Geometry: final body of the model. Coordinates: model frame, mm. Coordinates: 2 decimals unless noted, no trailing zeros. Write each loop counter-clockwise with the first axis right and the second up, starting at its lowest first coordinate (ties: lowest second). Pieces come first, ordered by that corner, then holes. Notation, with made-up numbers: (3.25, -31) -> (26.25, -31) arc R22 cw to (26.25, 6) -> close; hole circle Ø1 at (49.5, -17.5). An arc over 180 degrees is marked (long way). Answer as a JSON object with one key per item and string values. Group by question number.
```python
from build123d import *

# Parameters (mm, degrees)
SKETCH1_R           = 2.55
SKETCH1_R_2         = 4.5
SKETCH1_R_3         = 2.65
SKETCH1_W           = 44
SKETCH1_H           = 5
BOSS_EXTRUDE1_DEPTH = 5


with BuildPart() as part:
    # Sketch1 → Boss-Extrude1 (new body)
    with BuildSketch(Plane(origin=(0, 0, 0), x_dir=(1, 0, 0), z_dir=(0, 1, 0))):
        with BuildLine():
            Line((0, 0), (0, 33.5))
            ThreePointArc((0, 33.5), (-1.464466094, 37.035533906), (-5, 38.5))
            Line((-5, 38.5), (-31, 38.5))
            Line((-31, 38.5), (-31, 65))
            Line((-31, 65), (-564, 65))
            Line((-564, 65), (-564, -65))
            Line((-564, -65), (-524.5, -65))
            Line((-524.5, -65), (0, -65))
            Line((0, -65), (0, 0))
        make_face()
        with Locations(Location((-24.5, 33.5, 0), (0, 0, 270))):
            Circle(SKETCH1_R, mode=Mode.SUBTRACT)
        with Locations(Location((-24.5, -2.5, 0), (0, 0, 270))):
            Circle(SKETCH1_R, mode=Mode.SUBTRACT)
        with Locations(Location((-24.5, 15.5, 0), (0, 0, 270))):
            Circle(SKETCH1_R_2, mode=Mode.SUBTRACT)
        with Locations(Location((-531, -51, 0), (0, 0, 270))):
            Circle(SKETCH1_R_3, mode=Mode.SUBTRACT)
        with Locations(Location((-406, -51, 0), (0, 0, 270))):
            Circle(SKETCH1_R_3, mode=Mode.SUBTRACT)
        with Locations(Location((-281, -51, 0), (0, 0, 270))):
            Circle(SKETCH1_R_3, mode=Mode.SUBTRACT)
        with Locations(Location((-156, -51, 0), (0, 0, 270))):
            Circle(SKETCH1_R_3, mode=Mode.SUBTRACT)
        with Locations(Location((-31, -51, 0), (0, 0, 270))):
            Circle(SKETCH1_R_3, mode=Mode.SUBTRACT)
        with Locations((-472.510496642, 37)):
            Rectangle(SKETCH1_W, SKETCH1_H, mode=Mode.SUBTRACT)
        with Locations((-384.510496642, 37)):
            Rectangle(SKETCH1_W, SKETCH1_H, mode=Mode.SUBTRACT)
        with BuildLine():
            Line((-544.5, 36.05), (-524.5, 36.05))
            ThreePointArc((-524.5, 36.05), (-521.95, 33.5), (-524.5, 30.95))
            Line((-524.5, 30.95), (-544.5, 30.95))
            ThreePointArc((-544.5, 30.95), (-547.05, 33.5), (-544.5, 36.05))
        make_face(mode=Mode.SUBTRACT)
        with BuildLine():
            Line((-524.5, 0.05), (-544.5, 0.05))
            ThreePointArc((-544.5, 0.05), (-547.05, -2.5), (-544.5, -5.05))
            Line((-544.5, -5.05), (-524.5, -5.05))
            ThreePointArc((-524.5, -5.05), (-521.95, -2.5), (-524.5, 0.05))
        make_face(mode=Mode.SUBTRACT)
        with Locations((-296.510496642, 37)):
            Rectangle(SKETCH1_W, SKETCH1_H, mode=Mode.SUBTRACT)
        with BuildLine():
            Line((-544.5, 20), (-524.5, 20))
            ThreePointArc((-524.5, 20), (-520, 15.5), (-524.5, 11))
            Line((-524.5, 11), (-544.5, 11))
            ThreePointArc((-544.5, 11), (-549, 15.5), (-544.5, 20))
        make_face(mode=Mode.SUBTRACT)
        with Locations((-208.510496642, 37)):
            Rectangle(SKETCH1_W, SKETCH1_H, mode=Mode.SUBTRACT)
        with Locations((-120.510496642, 37)):
            Rectangle(SKETCH1_W, SKETCH1_H, mode=Mode.SUBTRACT)
    extrude(amount=BOSS_EXTRUDE1_DEPTH)


solid = part.part
```
Item 1: Mould query, pull axis X, two halves, no side actions, for faces 1 (the flat face through (-286, 5, -1)), 2 (the cylindrical face through (-21.46, 2.46, -18.82)). Classes: +X half, -X half, draft (parallel to the pull), parting line (faces both ways), or undercut.
Item 2: Section A-A on x = -218. Output: boundary loops of the cut face in (y, z).
Item 3: Contact query for flat-ended pins moving along their axis: pin 1 (1.5 mm diameter, centred on y = 2.5, z = -38, fed in from +X); pin 2 (3 mm diameter, centred on x = -24.5, z = 2.5, fed in from +Y) (3 decimals). Output: stop coordinate, or through.
Item 4: Section C-C on z = -49. Output: boundary loops of the cut face in (x, y), then the cut area to 4 significant figures.
Item 5: Ray query, L1, parallel to X at y = 3.7, z = -33.5; L2, parallel to Z at x = -406, y = 2.8; L3, parallel to X at y = 3.6, z = 51. Return the intervals inside material, ascending. Write a range as [from, to].
Item 6: Section B-B on y = 4.05. Give the number of separate pieces and of enclosed holes in the cut face, then the cut area to 3 significant figures.
Answer sheet:
{
 "1": {"face 1": "draft", "face 2": "undercut"},
 "2": {"outline": "(0, -65) -> (5, -65) -> (5, -39.5) -> (0, -39.5) -> close; (0, -34.5) -> (5, -34.5) -> (5, 65) -> (0, 65) -> close"},
 "3": {"pin 1": "stops at x = -1.69", "pin 2": "passes through"},
 "4": {"outline": "(-564, 0) -> (-31, 0) -> (-31, 5) -> (-564, 5) -> close", "area": "2,665 mm^2"},
 "5": {"L1": "x = [-564, -547.05], [-521.95, -27.05], [-21.95, 0]", "L2": "z = [-65, -39.5], [-34.5, 48.35], [53.65, 65]", "L3": "x = [-564, -533.65], [-528.35, -408.65], [-403.35, -283.65], [-278.35, -158.65], [-153.35, -33.65], [-28.35, 0]"},
 "6": {"separate pieces": "1", "enclosed holes": "16", "area": "70,700 mm^2"}
}
